Here's how the part is built. I have some questions about the finished solid (model axes, mm). Face numbers are marked on the shaded views. A direction names the side the tool comes from. Round coordinates to 2 decimals unless told otherwise and drop trailing zeros. Loops run counter-clockwise (first coordinate to the right, second up) from the corner with the lowest first, then second, coordinate; pieces in that order, holes last. Notation, with made-up numbers: M -13.5,7 L 45.5,7 A35 cw 45.5,45 Z; hole C 25,-17.5 d7. An arc over 180 degrees is marked long. Answer as CSV lines item,"result".
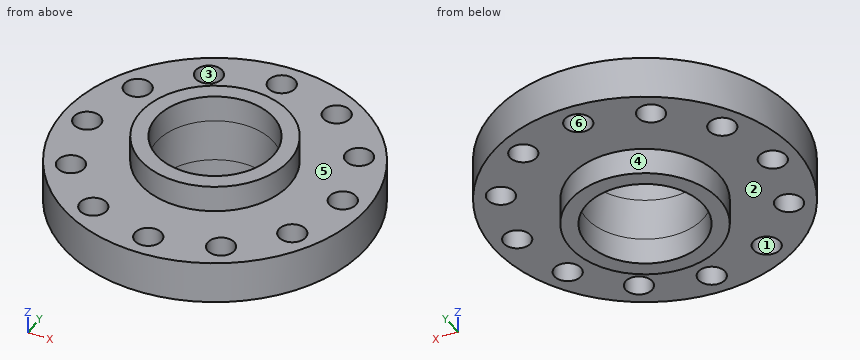
```python
from build123d import *
from build123d.topology import SkipClean

# Parameters (mm, degrees)
SKETCH1_R           = 28.4
SKETCH1_R_2         = 11
BOSS_EXTRUDE1_DEPTH = 8
BOSS_EXTRUDE2_START = 5
SKETCH2_R           = 14
SKETCH2_R_2         = 11
BOSS_EXTRUDE2_DEPTH = 5
SKETCH3_R           = 2.5
CUT_EXTRUDE1_DEPTH  = 43.215163153
CIRPATTERN1_COUNT   = 12
SCALE1_SCALE        = 0.24


with BuildPart() as part:
    # Sketch1 → Boss-Extrude1 (new body)
    with BuildSketch(Plane.XY):
        Circle(SKETCH1_R)
        Circle(SKETCH1_R_2, mode=Mode.SUBTRACT)
    extrude(amount=BOSS_EXTRUDE1_DEPTH)

    # Sketch2 → Boss-Extrude2 (add)
    with SkipClean():  # the faces are left unmerged after this step: merging them gives an invalid solid
        with BuildSketch(Plane(origin=(0, 0, 0), x_dir=(-1, 0, 0), z_dir=(0, 0, -1)).offset(BOSS_EXTRUDE2_START)):
            with Locations(Location((0, 0, 0), (0, 0, 180))):
                Circle(SKETCH2_R)
            Circle(SKETCH2_R_2, mode=Mode.SUBTRACT)
        boss_extrude2 = extrude(amount=-BOSS_EXTRUDE2_DEPTH)

    # Mirror1: Boss-Extrude2 across plane
    add(boss_extrude2.mirror(Plane.XY.offset(4)))

    # Sketch3 → Cut-Extrude1 (cut, through all)
    with BuildSketch(Plane(origin=(0, 0, 0), x_dir=(-1, 0, 0), z_dir=(0, 0, -1))):
        with Locations((11.9, 20.61140461)):
            Circle(SKETCH3_R)
    cut_extrude1 = extrude(amount=-CUT_EXTRUDE1_DEPTH, mode=Mode.SUBTRACT)

    # CirPattern1: Cut-Extrude1 ×12 about axis
    cirpattern1_axis = Axis((0, 0, 0), (0, 0, 1))
    for i in range(1, CIRPATTERN1_COUNT):
        add(cut_extrude1.rotate(cirpattern1_axis, i * 360 / CIRPATTERN1_COUNT), mode=Mode.SUBTRACT)


with BuildPart() as part_1:
    # Scale1: scaled about (0, 0, 4)
    add(part.part.scale(SCALE1_SCALE).moved(Location((0, 0, 3.04))))


solid = part_1.part
```
1. Which directions (+Z, -Z, +X, -X, +Y, -Y) give clear straight access to the entire face, cutting with the end or side of a thin tool? Please do the marked faces 5 and 6.
Evaluation:
face 5,"+Z"
face 6,"+Z, -Z"
2. If I drill on line 1 (X direction, y = 4.75, z = 4.7); line 2 (Y direction, x = -2.75, z = 4.5); line 3 (Z direction, x = -4.75, y = -2), over which ranges is the centre line in solid material (lowest first)? Write a range as [from, to].
Evaluation:
line 1,"x = [-4.89, -3.42], [-2.29, 2.29], [3.42, 4.89]"
line 2,"y = [-6.24, -5.54], [-4.36, 4.36], [5.54, 6.24]"
line 3,"z = [3.04, 4.96]"
3. We'd pull the mould along Y, two halves only. Please class the marked faces 1, 2, 3 and 4: pulls with the +Y half, pulls with the -Y half, needs draft (parallel to the pull), parting line crosses it, or undercut.
Evaluation:
face 1,"undercut"
face 2,"needs draft"
face 3,"undercut"
face 4,"parting line crosses it"
4. I want a section at D-D, the plane z = 4.05. Count the separate pieces of the cut face and the enclosed holes in it, and give its area (3 significant figures).
Evaluation:
separate pieces,"1"
enclosed holes,"13"
area,"110 mm²"
5. For P1, Ø1.1, axis at x = -5.712, y = 0, coming from the -Z side; P2, Ø1.6, axis at x = -4.95, y = -2.86, coming from the +Z side; P3, Ø1.9, axis at x = 0, y = 5.712, coming from the -Z side, each with a flat end and sliding along its axis, tell me the tip position at first contact or that it passes through.
Evaluation:
P1,"passes through"
P2,"stops at z = 4.96"
P3,"stops at z = 3.04"
6. I want a section at C-C, the plane x = -2. Please give me the cut outline in (y, z), and give its area (3 significant figures).
Evaluation:
outline,"M -6.52,3.04 L -2.7,3.04 L -2.7,1.84 L -1.72,1.84 L -1.72,6.16 L -2.7,6.16 L -2.7,4.96 L -6.52,4.96 Z; M 1.72,1.84 L 2.7,1.84 L 2.7,3.04 L 6.52,3.04 L 6.52,4.96 L 2.7,4.96 L 2.7,6.16 L 1.72,6.16 Z"
area,"23.1 mm²"
7. I want a section at A-A, the plane y = 0. Please give me the cut outline in (x, z), and give its area (3 significant figures).
Evaluation:
outline,"M -6.82,3.04 L -6.31,3.04 L -6.31,4.96 L -6.82,4.96 Z; M -5.11,3.04 L -3.36,3.04 L -3.36,1.84 L -2.64,1.84 L -2.64,6.16 L -3.36,6.16 L -3.36,4.96 L -5.11,4.96 Z; M 2.64,1.84 L 3.36,1.84 L 3.36,3.04 L 5.11,3.04 L 5.11,4.96 L 3.36,4.96 L 3.36,6.16 L 2.64,6.16 Z; M 6.31,3.04 L 6.82,3.04 L 6.82,4.96 L 6.31,4.96 Z"
area,"14.9 mm²"
